Geometry: final body of the model. Coordinates: model frame, mm. A direction names the side the tool comes from. Coordinates: 2 decimals unless noted, no trailing zeros. Order: outer loops, then holes, each group sorted by start corner. A loop starts at its lowest first (then second) coordinate and runs counter-clockwise, first axis right, second up. Notation, with made-up numbers: M 14,53.5 L 19,53.5 A23 ccw 19,75.5 Z; hole C -19,4.5 d6. An arc over 180 degrees is marked long. Use CSV: the item, a comma, the result in double quotes. Start each with the question number.
Q1. Section query A-A, the plane x = 153. Output: boundary loops of the cut face in (y, z), and give its area (3 significant figures).
Q2. First-contact query: P1, Ø3, axis at y = -2, z = -2, coming from the +X side; P2, Ø6, axis at x = 219.5, y = 4, coming from the -Z side; P3, Ø5, axis at x = 167, y = -3, coming from the -Z side. Flat tips, straight axial feed; report the tip coordinate or a pass-through.
Q3. Access query for faces 1 (the face through (275, 0, 0)), 2 (the face through (290, 2, 5)). Directions: +Z, -Z, +X, -X, +Y, -Y. A direction counts if a zero-diameter tool reaches every point of the face in a straight line with its end or side. Return the directions, or none.
Q4. Ray query, probe 1 along X at (y, z) = (0, 3.75); probe 2 along X at (y, z) = (0, 5.75); probe 3 along Y at (x, z) = (33.75, 4.75). Return the intervals inside material, ascending.
Q5. Mould query, pull axis Y, two halves, no side actions, for faces 3 (the face through (282.6, -4.88, 1.08)), 4 (the face through (142.97, -2.17, 9.76)), 5 (the face through (0, 0, 0)). Classes: +Y half, -Y half, draft (parallel to the pull), parting line (faces both ways), or undercut.
Autodesk Inventor part; units mm, degrees
ref_plane "YZ Plane" through (0, 0, 0) normal (1, 0, 0) x (0, 1, 0)
ref_plane "XZ Plane" through (0, 0, 0) normal (0, 1, 0) x (-1, 0, 0)
ref_plane "XY Plane" through (0, 0, 0) normal (0, 0, 1) x (1, 0, 0)
sketch "Boceto1" plane through (0, 0, 0) normal (0, 0, 1) x (1, 0, 0)
  line L0 (0, 0) -> (290, 0)
  line L1 (290, 0) -> (290, 10)
  line L2 (0, 10) -> (0, 0)
  line L3 (290, 10) -> (0, 10)
  dimension "d0" = 10
  dimension "d1" = 290
revolve "Revolución1" add sketch "Boceto1" angle 360 about axis through (0, 0, 0) along (1, 0, 0)
sketch "Boceto3" plane through (290, 0, 0) normal (1, 0, 0) x (0, 0, -1)
  circle A0 centre (0, 0) radius 5
  dimension "d10" = 10
extrude "Extrusión2" cut sketch "Boceto3" against normal blind 15
thread "Rosca1"
sketch "Sketch4" plane through (0, 0, 0) normal (0, 0, 1) x (1, 0, 0)
  circle A0 centre (33.75, 0) radius 1.5
  line L0 (0, -10) -> (0, 10)
  point P0 (0, 0)
  dimension "d15" = 3
  dimension "d16" = 33.75
extrude "Extrusion3" cut sketch "Sketch4" along normal blind 33.75
thread "Thread2"
equation "\"d17\" = d16"
properties part number "Eje_Base" material "Acero, carbono"
Responses:
1,outline,"C 0,0 d20"
1,area,"314 mm²"
2,P1,"stops at x = 275"
2,P2,"stops at z = -9.95"
2,P3,"stops at z = -9.99"
3,face 1,"+X"
3,face 2,"+Z, -Z, +X, +Y, -Y"
4,probe 1,"x = 0 to 32.25, 35.25 to 275"
4,probe 2,"x = 0 to 32.25, 35.25 to 290"
4,probe 3,"y = -8.8 to -1.5, 1.5 to 8.8"
5,face 3,"undercut"
5,face 4,"parting line"
5,face 5,"draft"
